Part model, mm, in its own coordinate system. Face numbers are marked on the shaded views. A direction names the side the tool comes from. Round coordinates to 2 decimals unless told otherwise and drop trailing zeros. Loops run counter-clockwise (first coordinate to the right, second up) from the corner with the lowest first, then second, coordinate; pieces in that order, holes last.
from build123d import *

# Parameters (mm, degrees)
SKETCH1_R           = 7
BOSS_EXTRUDE1_DEPTH = 3
SKETCH1_3_R         = 4
BOSS_EXTRUDE2_DEPTH = 45
CHAMFER1_SIZE       = 1
CUT_EXTRUDE1_REACH  = 48.851
SKETCH2_R           = 0.95


with BuildPart() as part:
    # Sketch1 → Boss-Extrude1 (new body)
    with BuildSketch(Plane(origin=(0, 0, 0), x_dir=(1, 0, 0), z_dir=(0, 1, 0))):
        with Locations(Location((0, 0, 0), (0, 0, 270))):
            Circle(SKETCH1_R)
    extrude(amount=-BOSS_EXTRUDE1_DEPTH)

    # Sketch1_3 → Boss-Extrude2 (add)
    with BuildSketch(Plane(origin=(0, 0, 0), x_dir=(1, 0, 0), z_dir=(0, 1, 0))):
        with Locations(Location((0, 0, 0), (0, 0, 90))):
            Circle(SKETCH1_3_R)
    extrude(amount=BOSS_EXTRUDE2_DEPTH)

    # Chamfer1
    chamfer1_edges = [part.edges().sort_by_distance(p)[0] for p in [
        (0, -3, -7),
    ]]
    chamfer(chamfer1_edges, length=CHAMFER1_SIZE)

    # Sketch2 → Cut-Extrude1 (cut, up to next)
    with BuildSketch(Plane.XY.offset(4), mode=Mode.PRIVATE) as cut_extrude1_sk1:
        with Locations((0, 43)):
            Circle(SKETCH2_R)
    cut_extrude1_tool1 = extrude(cut_extrude1_sk1.sketch, amount=-CUT_EXTRUDE1_REACH, mode=Mode.PRIVATE) & part.part
    add(cut_extrude1_tool1.solids().sort_by_distance((0, 43, 4))[0], mode=Mode.SUBTRACT)


solid = part.part
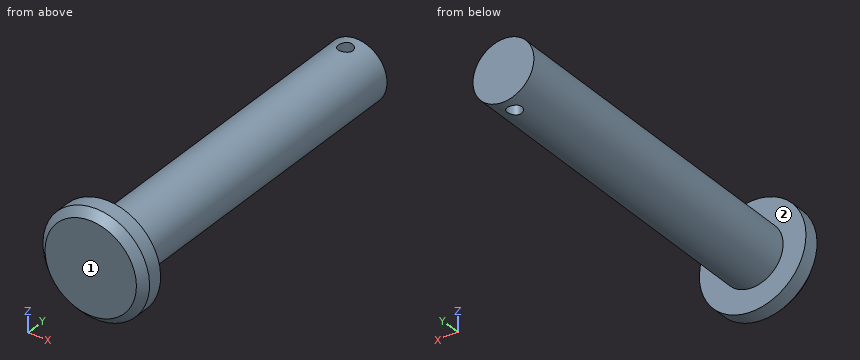
1) Slice it at D-D, the plane y = 43. Give the cut face in (x, z).
Values:
outline: (-0.95, -3.89) - (-0.95, 3.89) arc R4 ccw to start; (0.95, -3.89) arc R4 ccw to (0.95, 3.89) - close
2) Drop flat-ended pins along their axis: pin 1 Ø1.1 at (x, y) = (0, 43) entering from +Z; pin 2 Ø8 at (x, z) = (-4.5, -2.5) entering from +Y; pin 3 Ø5 at (y, z) = (32.5, 2.5) entering from +X. Give the stop position or say it passes through.
Values:
pin 1: passes through
pin 2: stops at y = 45
pin 3: stops at x = 4
3) Tool access for the marked faces 1 and 2: list every direction of +Z, -Z, +X, -X, +Y, -Y with a clear straight run to the whole face (end or side of a thin tool).
Values:
face 1: +Z, -Z, +X, -X, -Y
face 2: +Y
4) Slice it at A-A, the plane x = 0. Give the cut face in (y, z), then the cut area to 3 significant figures.
Values:
outline: (-3, -6) - (-2, -7) - (0, -7) - (0, -4) - (42.05, -4) - (42.05, 4) - (0, 4) - (0, 7) - (-2, 7) - (-3, 6) - close; (43.95, -4) - (45, -4) - (45, 4) - (43.95, 4) - close
area: 386 mm2
5) Slice it at B-B, the plane z = 0. Give the cut face in (x, y), then the cut area to 3 significant figures.
Values:
outline: (-7, -2) - (-6, -3) - (6, -3) - (7, -2) - (7, 0) - (4, 0) - (4, 45) - (-4, 45) - (-4, 0) - (-7, 0) - close; hole circle Ø1.9 at (0, 43)
area: 398 mm2
6) Wall check: line 1 along Y through (x, z) = (0, 1); line 2 along X through (y, z) = (43, 1); line 3 along Y through (x, z) = (4, 2). Give the ranges that are in metal, low to high.
Values:
line 1: y = -3 to 42.05, 43.95 to 45
line 2: x = -3.87 to -0.95, 0.95 to 3.87
line 3: y = -3 to 0
7) Slice it at C-C, the plane y = 22. Give the cut face in (x, z), then the cut area to 3 significant figures.
Values:
outline: circle Ø8 at (0, 0)
area: 50.3 mm2
